from build123d import *

# Parameters (mm, degrees)
SKETCH1_R           = 5
BOSS_EXTRUDE1_DEPTH = 1
SKETCH2_R           = 5
BOSS_EXTRUDE2_DEPTH = 5
SKETCH3_R           = 1.65
CUT_EXTRUDE3_DEPTH  = 3
CHAMFER3_SIZE       = 3.3
CHAMFER4_SIZE       = 0.5
SKETCH4_W           = 1
SKETCH4_H           = 3.5
CUT_EXTRUDE4_DEPTH  = 1
FILLET1_R           = 0.5


with BuildPart() as part:
    # Sketch1 → Boss-Extrude1 (new body)
    with BuildSketch(Plane(origin=(0, 0, 0), x_dir=(1, 0, 0), z_dir=(0, 1, 0))):
        with Locations(Location((0, 0, 0), (0, 0, 270))):
            Circle(SKETCH1_R)
    extrude(amount=BOSS_EXTRUDE1_DEPTH)

    # Sketch2 → Boss-Extrude2 (add)
    with BuildSketch(Plane(origin=(0, 1, 0), x_dir=(1, 0, 0), z_dir=(0, 1, 0))):
        with Locations(Location((0, 0, 0), (0, 0, 270))):
            Circle(SKETCH2_R)
    extrude(amount=BOSS_EXTRUDE2_DEPTH)

    # Sketch3 → Cut-Extrude3 (cut)
    with BuildSketch(Plane(origin=(0, 6, 0), x_dir=(1, 0, 0), z_dir=(0, 1, 0))):
        with Locations(Location((0, 0, 0), (0, 0, 270))):
            Circle(SKETCH3_R)
    extrude(amount=-CUT_EXTRUDE3_DEPTH, mode=Mode.SUBTRACT)

    # Chamfer3
    chamfer3_edges = [part.edges().sort_by_distance(p)[0] for p in [
        (0, 6, -5),
    ]]
    chamfer(chamfer3_edges, length=CHAMFER3_SIZE)

    # Chamfer4
    chamfer4_edges = [part.edges().sort_by_distance(p)[0] for p in [
        (0, 0, -5),
    ]]
    chamfer(chamfer4_edges, length=CHAMFER4_SIZE)

    # Sketch4 → Cut-Extrude4 (cut)
    with BuildSketch(Plane.XZ):
        with BuildLine():
            Line((-2.007517527, -2.867032155), (-1.433941091, -2.047880111))
            ThreePointArc((-1.433941091, -2.047880111), (0, 2.5), (1.433941091, -2.047880111))
            Line((1.433941091, -2.047880111), (2.007517527, -2.867032155))
            ThreePointArc((2.007517527, -2.867032155), (0, 3.5), (-2.007517527, -2.867032155))
        make_face()
        with Locations((0, -1.75)):
            Rectangle(SKETCH4_W, SKETCH4_H)
    extrude(amount=-CUT_EXTRUDE4_DEPTH, mode=Mode.SUBTRACT)

    # Fillet1
    fillet1_edges = [part.edges().sort_by_distance(p)[0] for p in [
        (1.433941091, 0.5, -2.047880111),
        (2.007517527, 0.5, -2.867032155),
        (0.5, 0.5, -3.5),
        (0.5, 0.5, 0),
        (-0.5, 0.5, 0),
        (-0.5, 0.5, -3.5),
        (-1.433941091, 0.5, -2.047880111),
        (-2.007517527, 0.5, -2.867032155),
    ]]
    fillet(fillet1_edges, radius=FILLET1_R - 0.0001)  # a hair under: the kernel refuses the full size


solid = part.part
The listing builds one solid part. Answer for the finished solid, in the listing's coordinates (mm). A direction names the side the tool comes from. Give positions to 0.01 mm unless a question says otherwise; leave off trailing zeros. Write each loop counter-clockwise with the first axis right and the second up, starting at its lowest first coordinate (ties: lowest second). Pieces come first, ordered by that corner, then holes.
1) Find the intervals of material crossed by L1, parallel to X at y = 3.8, z = 0; L2, parallel to Z at x = 1, y = 4.2; L3, parallel to Y at x = 0, z = -1.25, in increasing order.
2) Section A-A (y = 3.4) is taken. Write down the section's boundary in (x, z).
3) A tool of negligible diameter and unlimited length cuts with its end or side. For faces 4 (the face through (-1, 4.52, -1.31)), 5 (the face through (0.1, 0.5, 3.5)), 6 (the face through (-4.88, 1.58, -1.08)), from which of +Z, -Z, +X, -X, +Y, -Y can it reach the whole face along a straight path? Write none if from no direction.
4) For a pull along Z with two mould halves and no side action, classify faces 1 (the face through (-1, 0, 0)), 2 (the face through (0.6, 5.8, 1.8)), 3 (the face through (-1.1, 1, 2.5)) as pulls with the +Z half, pulls with the -Z half, needs draft (parallel to the pull), parting line crosses it, or undercut.
5) Given P1, Ø1.1, axis at y = 0.5, z = -2, coming from the -X side; P2, Ø1.5, axis at x = -2, y = 1, coming from the +Z side; P3, Ø3, axis at x = -3, z = 2.5, coming from the +Y side, each flat-ended and moving along its own axis, determine where each tip first touches the part or whether it passes through.
6) Section B-B (y = 4.25) is taken. Write down the section's boundary in (x, z), and give its area (3 significant figures).
Response:
1. L1: x = -3.9 to -1.65, 1.65 to 3.9
1. L2: z = -3.35 to -1.31, 1.31 to 3.35
1. L3: y = 1 to 3
2. outline: circle Ø8.6 at (0, 0); hole circle Ø3.3 at (0, 0)
3. face 4: +Y
3. face 5: -Y
3. face 6: +Y, -Y
4. face 1: needs draft
4. face 2: parting line crosses it
4. face 3: undercut
5. P1: stops at x = -4.79
5. P2: stops at z = 4.84
5. P3: stops at y = 5.29
6. outline: circle Ø6.9 at (0, 0); hole circle Ø3.3 at (0, 0)
6. area: 28.8 mm2
